from build123d import *

# Parameters (mm, degrees)
SKETCH2_W           = 40
SKETCH2_H           = 20
SKETCH2_R           = 2
BOSS_EXTRUDE1_DEPTH = 3.5
SKETCH3_W           = 24
SKETCH3_H           = 20
BOSS_EXTRUDE2_DEPTH = 10.5
SKETCH4_W           = 18
SKETCH4_H           = 17
CUT_EXTRUDE2_DEPTH  = 10
SKETCH5_R           = 3.25
CUT_EXTRUDE3_DEPTH  = 15


with BuildPart() as part:
    # Sketch2 → Boss-Extrude1 (new body)
    with BuildSketch(Plane.XY):
        with Locations((-41.200062639, 6.409268178)):
            Rectangle(SKETCH2_W, SKETCH2_H)
        with Locations((-57.200062639, 6.409268178)):
            Circle(SKETCH2_R, mode=Mode.SUBTRACT)
        with Locations((-25.200062639, 6.409268178)):
            Circle(SKETCH2_R, mode=Mode.SUBTRACT)
    extrude(amount=BOSS_EXTRUDE1_DEPTH)

    # Sketch3 → Boss-Extrude2 (add)
    with BuildSketch(Plane.XY.offset(3.5)):
        with Locations((-41.200062639, 6.409268178)):
            Rectangle(SKETCH3_W, SKETCH3_H)
    extrude(amount=BOSS_EXTRUDE2_DEPTH)

    # Sketch4 → Cut-Extrude2 (cut)
    with BuildSketch(Plane(origin=(0, 0, 0), x_dir=(-1, 0, 0), z_dir=(0, 0, -1))):
        with Locations((41.200062639, 6.409268178)):
            Rectangle(SKETCH4_W, SKETCH4_H)
    extrude(amount=-CUT_EXTRUDE2_DEPTH, mode=Mode.SUBTRACT)

    # Sketch5 → Cut-Extrude3 (cut, through all)
    with BuildSketch(Plane.XY.offset(14)):
        with Locations((-41.200062639, 6.409268178)):
            Circle(SKETCH5_R)
    extrude(amount=-CUT_EXTRUDE3_DEPTH, mode=Mode.SUBTRACT)


solid = part.part
Could you check a few things on this model? Use its own coordinates, in mm. A direction names the side the tool comes from. Round coordinates to 2 decimals unless told otherwise and drop trailing zeros. Order: outer loops, then holes, each group sorted by start corner. A loop starts at its lowest first (then second) coordinate and runs counter-clockwise, first axis right, second up.
(1) Which directions (+Z, -Z, +X, -X, +Y, -Y) give clear straight access to the entire face, cutting with the end or side of a thin tool? Please do faces 1 (the flat face through (-53.2, 6, 9)), 2 (the flat face through (-44, 4, 14)), 3 (the flat face through (-25, 9, 3.5)), 4 (the flat face through (-50.2, 6, 5)).
Response values:
face 1: +Z, -X, +Y, -Y
face 2: +Z, +X, -X, +Y, -Y
face 3: +Z, +X, +Y, -Y
face 4: -Z
(2) Imagine slicing it at D-D (y = 9). Write out the boundary of the cut face in (x, z).
Response values:
outline: (-61.2, 0) - (-50.2, 0) - (-50.2, 10) - (-43.16, 10) - (-43.16, 14) - (-53.2, 14) - (-53.2, 3.5) - (-61.2, 3.5) - close; (-39.24, 10) - (-32.2, 10) - (-32.2, 0) - (-21.2, 0) - (-21.2, 3.5) - (-29.2, 3.5) - (-29.2, 14) - (-39.24, 14) - close
(3) Please list where these lines run through material, in increasing order: line 1 along X through (y, z) = (8.75, 6); line 2 along Y through (x, z) = (-46, 1.5); line 3 along X through (y, z) = (2.75, 2.75).
Response values:
line 1: x = -53.2 to -50.2, -32.2 to -29.2
line 2: y = -3.59 to -2.09, 14.91 to 16.41
line 3: x = -61.2 to -50.2, -32.2 to -21.2
(4) Imagine slicing it at C-C (z = 6.5). Write out the boundary of the cut face in (x, y), plus the area to 3 significant figures.
Response values:
outline: (-53.2, -3.59) - (-29.2, -3.59) - (-29.2, 16.41) - (-53.2, 16.41) - close; hole (-50.2, -2.09) - (-32.2, -2.09) - (-32.2, 14.91) - (-50.2, 14.91) - close
area: 174 mm2
(5) I'm going to push flat-ended pins straight in: pin 1 (5 mm diameter, centred on x = -57.2, y = 6.41, fed in from +Z); pin 2 (5 mm diameter, centred on x = -38, y = 9.5, fed in from -Z); pin 3 (2 mm diameter, centred on y = 4, z = 7.5, fed in from -X). Where does each tip first touch, or does it pass through?
Response values:
pin 1: stops at z = 3.5
pin 2: stops at z = 10
pin 3: stops at x = -53.2
(6) Imagine slicing it at B-B (x = -33). Write out the boundary of the cut face in (y, z).
Response values:
outline: (-3.59, 0) - (-2.09, 0) - (-2.09, 10) - (14.91, 10) - (14.91, 0) - (16.41, 0) - (16.41, 14) - (-3.59, 14) - close
(7) If we mould it in two halves opening along X, with no side actions, what happens to faces 5 (the flat face through (-61.2, 6, 2)), 6 (the cylindrical face through (-23.353, 5.643, 1.726)), 7 (the flat face through (-41, -3.591, 5))? For each: released by +X, released by -X, zero draft, split by the parting line, or undercut.
Response values:
face 5: released by -X
face 6: undercut
face 7: zero draft
(8) Imagine slicing it at A-A (y = 5.5). Write out the boundary of the cut face in (x, z).
Response values:
outline: (-61.2, 0) - (-58.98, 0) - (-58.98, 3.5) - (-61.2, 3.5) - close; (-55.42, 0) - (-50.2, 0) - (-50.2, 10) - (-44.32, 10) - (-44.32, 14) - (-53.2, 14) - (-53.2, 3.5) - (-55.42, 3.5) - close; (-38.08, 10) - (-32.2, 10) - (-32.2, 0) - (-26.98, 0) - (-26.98, 3.5) - (-29.2, 3.5) - (-29.2, 14) - (-38.08, 14) - close; (-23.42, 0) - (-21.2, 0) - (-21.2, 3.5) - (-23.42, 3.5) - close
